from build123d import *

# Parameters (mm, degrees)
SALIENTE_EXTRUIR1_DEPTH = 30
CROQUIS3_W              = 4.89350096
CROQUIS3_H              = 4.01782184
SALIENTE_EXTRUIR2_DEPTH = 3
SALIENTE_EXTRUIR3_DEPTH = 1


with BuildPart() as part:
    # Croquis1 → Saliente-Extruir1 (new body)
    with BuildSketch(Plane(origin=(0, 0, 0), x_dir=(1, 0, 0), z_dir=(0, 1, 0))):
        with BuildLine():
            Line((-6, 8), (6, 8))
            ThreePointArc((6, 8), (10.242640687, 6.242640687), (12, 2))
            Line((12, 2), (12, -2))
            ThreePointArc((12, -2), (10.242640687, -6.242640687), (6, -8))
            Line((6, -8), (-6, -8))
            ThreePointArc((-6, -8), (-10.242640687, -6.242640687), (-12, -2))
            Line((-12, -2), (-12, 2))
            ThreePointArc((-12, 2), (-10.242640687, 6.242640687), (-6, 8))
        make_face()
        with BuildLine():
            Line((-6, -5), (6, -5))
            ThreePointArc((6, -5), (8.121320344, -4.121320344), (9, -2))
            Line((9, -2), (9, 2))
            ThreePointArc((9, 2), (8.121320344, 4.121320344), (6, 5))
            Line((6, 5), (-6, 5))
            ThreePointArc((-6, 5), (-8.121320344, 4.121320344), (-9, 2))
            Line((-9, 2), (-9, -2))
            ThreePointArc((-9, -2), (-8.121320344, -4.121320344), (-6, -5))
        make_face(mode=Mode.SUBTRACT)
    extrude(amount=SALIENTE_EXTRUIR1_DEPTH)

    # Croquis3 → Saliente-Extruir2 (add)
    with BuildSketch(Plane(origin=(0, 0, -8), x_dir=(-1, 0, 0), z_dir=(0, 0, -1))):
        with Locations((0, 15)):
            Rectangle(CROQUIS3_W, CROQUIS3_H)
    extrude(amount=SALIENTE_EXTRUIR2_DEPTH)

    # Croquis5 → Saliente-Extruir3 (add)
    with BuildSketch(Plane.XZ):
        with BuildLine():
            Line((6, -5), (-6, -5))
            ThreePointArc((-6, -5), (-8.121320344, -4.121320344), (-9, -2))
            Line((-9, -2), (-9, 2))
            ThreePointArc((-9, 2), (-8.121320344, 4.121320344), (-6, 5))
            Line((-6, 5), (6, 5))
            ThreePointArc((6, 5), (8.121320344, 4.121320344), (9, 2))
            Line((9, 2), (9, -2))
            ThreePointArc((9, -2), (8.121320344, -4.121320344), (6, -5))
        make_face()
    extrude(amount=-SALIENTE_EXTRUIR3_DEPTH)


solid = part.part
Input: part model. Units: mm. Frame: model coordinates. A direction names the side the tool comes from. Coordinates: 2 decimals unless noted, no trailing zeros. Write each loop counter-clockwise with the first axis right and the second up, starting at its lowest first coordinate (ties: lowest second). Pieces come first, ordered by that corner, then holes. Notation, with made-up numbers: M 51,54 L 79,54 A10 ccw 79,68 Z; hole C 57.5,-39.75 d11. An arc over 180 degrees is marked long. Answer as a JSON object with one key per item and string values. Group by question number.
(1) Ray query, line 1 along Z through (x, y) = (1, 20.25); line 2 along Y through (x, z) = (-6.75, 2); line 3 along X through (y, z) = (9.25, 3.25). Return the intervals inside material, ascending. Write a range as [from, to].
(2) Section C-C on z = -4.5. Output: boundary loops of the cut face in (x, y).
(3) Section B-B on x = -1.75. Output: boundary loops of the cut face in (y, z).
(4) Section D-D on x = 7.5. Output: boundary loops of the cut face in (y, z), plus the area to 3 significant figures.
(5) Section A-A on y = 12. Output: boundary loops of the cut face in (x, z).
(6) Set-up query: faces 4 (the face through (2.447, 15, -9)), 5 (the face through (-8.14, 15.3, 4.1)), 6 (the face through (-10.289, 14.79, -6.196)), 7 (the face through (0, 17.009, -9)). Return all of +Z, -Z, +X, -X, +Y, -Y with unobstructed straight access to the full face (end or side cutting, diameter ignored); none if empty.
(7) Mould query, pull axis Z, two halves, no side actions, for faces 1 (the face through (0, 15, 8)), 2 (the face through (0, 1, 0)), 3 (the face through (0.2, 30, -5.4)). Classes: pulls with the +Z half, pulls with the -Z half, needs draft (parallel to the pull), parting line crosses it, or undercut.
(8) Contact query for flat-ended pins moving along their axis: P1, Ø3, axis at x = -2.5, z = 1.5, coming from the +Y side; P2, Ø1.5, axis at x = 0, z = -10, coming from the -Y side; P3, Ø3, axis at x = 8, y = 22.5, coming from the -Z side. Output: stop coordinate, or through.
Result set:
{
 "1": {"line 1": "z = [-8, -5], [5, 8]", "line 2": "y = [0, 1]", "line 3": "x = [-11.87, -8.73], [8.73, 11.87]"},
 "2": {"outline": "M -11.45,0 L 11.45,0 L 11.45,30 L 7.66,30 L 7.66,1 L -7.66,1 L -7.66,30 L -11.45,30 Z"},
 "3": {"outline": "M 0,-8 L 12.99,-8 L 12.99,-11 L 17.01,-11 L 17.01,-8 L 30,-8 L 30,-5 L 1,-5 L 1,5 L 30,5 L 30,8 L 0,8 Z"},
 "4": {"outline": "M 0,-7.81 L 30,-7.81 L 30,-4.6 L 1,-4.6 L 1,4.6 L 30,4.6 L 30,7.81 L 0,7.81 Z", "area": "202 mm2"},
 "5": {"outline": "M -12,-2 A6 ccw -6,-8 L 6,-8 A6 ccw 12,-2 L 12,2 A6 ccw 6,8 L -6,8 A6 ccw -12,2 Z; hole M -9,-2 A3 ccw -6,-5 L 6,-5 A3 ccw 9,-2 L 9,2 A3 ccw 6,5 L -6,5 A3 ccw -9,2 Z"},
 "6": {"face 4": "-Z, +X, +Y, -Y", "face 5": "+Y", "face 6": "-Z, -X, +Y, -Y", "face 7": "-Z, +X, -X, +Y"},
 "7": {"face 1": "pulls with the +Z half", "face 2": "undercut", "face 3": "needs draft"},
 "8": {"P1": "stops at y = 1", "P2": "stops at y = 12.99", "P3": "stops at z = -7.98"}
}
